For this review, take the finished solid that the model builds, in its own axes (mm). Face numbers are marked on the shaded views. A direction names the side the tool comes from. Coordinates: 2 decimals unless noted, no trailing zeros. Order: outer loops, then holes, each group sorted by start corner. A loop starts at its lowest first (then second) coordinate and runs counter-clockwise, first axis right, second up. Notation, with made-up numbers: M -16,-26 L 40,-26 A21 ccw 40,10 Z; hole C 52,32 d2. An arc over 180 degrees is marked long. Use one line per item in the form item = value. Start each with the question number.
```python
from build123d import *

# Parameters (mm, degrees)
BOSS_EXTRUDE1_DEPTH      = 8
SKETCH2_R                = 1.5
CUT_EXTRUDE1_DEPTH       = 10
SKETCH3_R                = 1.5
CUT_EXTRUDE2_DEPTH       = 10
BOSS_EXTRUDE3_DEPTH      = 30
BOSS_EXTRUDE3_DEPTH_BACK = 8
SKETCH6_W                = 20
SKETCH6_H                = 10
FILLET3_R                = 12
SKETCH7_W                = 20
SKETCH7_H                = 30
BOSS_EXTRUDE4_DEPTH      = 2
CUT_EXTRUDE3_DEPTH       = 10
SKETCH9_R                = 5.5
CUT_EXTRUDE4_DEPTH       = 10
FILLET4_R                = 5
FILLET5_R                = 2
CUT_EXTRUDE5_DEPTH       = 10
SKETCH11_W               = 20
SKETCH11_H               = 3
CUT_EXTRUDE6_DEPTH       = 15
FILLET6_R                = 2


with BuildPart() as part:
    # Sketch1 → Boss-Extrude1 (new body)
    with BuildSketch(Plane.XY):
        with BuildLine():
            Line((-25, 10), (40, 10))
            ThreePointArc((40, 10), (50, 0), (40, -10))
            Line((40, -10), (-25, -10))
            Line((-25, -10), (-25, 10))
        make_face()
    extrude(amount=BOSS_EXTRUDE1_DEPTH)

    # Sketch2 → Cut-Extrude1 (cut)
    with BuildSketch(Plane.XY.offset(8)):
        with Locations((40, 0)):
            Circle(SKETCH2_R)
    extrude(amount=-CUT_EXTRUDE1_DEPTH, mode=Mode.SUBTRACT)

    # Sketch3 → Cut-Extrude2 (cut)
    with BuildSketch(Plane(origin=(0, 0, 0), x_dir=(-1, 0, 0), z_dir=(0, 0, -1))):
        with Locations((-15, 0)):
            Circle(SKETCH3_R)
    extrude(amount=-CUT_EXTRUDE2_DEPTH, mode=Mode.SUBTRACT)

    # Sketch6 → Boss-Extrude3 (add, two sides: drawn at the far end of the back side and taken through both)
    with BuildSketch(Plane(origin=(0, 0, 0), x_dir=(-1, 0, 0), z_dir=(0, 0, -1)).offset(-BOSS_EXTRUDE3_DEPTH_BACK)):
        with Locations((15, -15)):
            Rectangle(SKETCH6_W, SKETCH6_H)
    extrude(amount=BOSS_EXTRUDE3_DEPTH + BOSS_EXTRUDE3_DEPTH_BACK)

    # Fillet3
    # the kernel refuses this fillet: 12 mm, written as the material it adds along each edge
    with BuildSketch(Plane(origin=(-5, -10, 8), x_dir=(0, -1, 0), z_dir=(0, 0, -1))) as fillet3_piece_1:
        with BuildLine():
            CenterArc((12, -11.832159566), FILLET3_R, 99.594068227, 80.405931773)
            Line((0, -11.832159566), (0, 0))
            Line((0, 0), (10, 0))
        make_face()
    extrude(amount=8)

    # Sketch7 → Boss-Extrude4 (add)
    with BuildSketch(Plane(origin=(0, -10, 0), x_dir=(1, 0, 0), z_dir=(0, 1, 0))):
        with Locations((-15, 15)):
            Rectangle(SKETCH7_W, SKETCH7_H)
    extrude(amount=BOSS_EXTRUDE4_DEPTH)

    # Sketch8 → Cut-Extrude3 (cut)
    with BuildSketch(Plane.XZ.offset(20)):
        Polygon((-12.092828782, -7.012612723), (-20.463694682, -8.488622233), (-23.370865901, -16.47600951), (-17.907171218, -22.987387277), (-9.536305318, -21.511377767), (-6.629134099, -13.52399049), align=None)
    extrude(amount=-CUT_EXTRUDE3_DEPTH, mode=Mode.SUBTRACT)

    # Sketch9 → Cut-Extrude4 (cut)
    with BuildSketch(Plane.XZ.offset(10)):
        with Locations(Location((-15, -15, 0), (0, 0, 270))):
            Circle(SKETCH9_R)
    extrude(amount=-CUT_EXTRUDE4_DEPTH, mode=Mode.SUBTRACT)

    # Fillet4
    # the kernel refuses this fillet: 5 mm, written as the material it adds along each edge
    with BuildSketch(Plane(origin=(-5, -20, 0), x_dir=(1, 0, 0), z_dir=(0, 1, 0))) as fillet4_piece_1_section:
        with BuildLine():
            CenterArc((FILLET4_R, FILLET4_R), FILLET4_R, 180, 90)
            Line((0, FILLET4_R), (0, 0))
            Line((0, 0), (FILLET4_R, 0))
        make_face()
    fillet4_piece_1 = extrude(amount=12, mode=Mode.PRIVATE)
    fillet4_piece_1 = fillet4_piece_1 - Plane(origin=(6.832159566, -22, 0), x_dir=(0, -1, 0), z_dir=(0, 0, 1)) * Cylinder(12, 44, mode=Mode.PRIVATE)
    add(fillet4_piece_1)
    with BuildSketch(Plane(origin=(-25, -8, 0), x_dir=(0, 1, 0), z_dir=(1, 0, 0))) as fillet4_piece_2:
        with BuildLine():
            CenterArc((FILLET4_R, -FILLET4_R), FILLET4_R, 90, 90)
            Line((0, -FILLET4_R), (0, 0))
            Line((0, 0), (FILLET4_R, 0))
        make_face()
    extrude(amount=20)
    with BuildSketch(Plane(origin=(-5, -20, 0), x_dir=(1, 0, 0), z_dir=(0, 1, 0))) as fillet4_piece_3a_section:
        with BuildLine():
            CenterArc((FILLET4_R, FILLET4_R), FILLET4_R, 180, 90)
            Line((0, FILLET4_R), (0, 0))
            Line((0, 0), (FILLET4_R, 0))
        make_face()
    fillet4_piece_3a = extrude(amount=24.5, mode=Mode.PRIVATE)
    fillet4_piece_3a = split(fillet4_piece_3a, bisect_by=Plane(origin=(-5, -8, 0), z_dir=(0, 1, 0)), keep=Keep.TOP, mode=Mode.PRIVATE)
    with BuildSketch(Plane(origin=(-25, -8, 0), x_dir=(0, 1, 0), z_dir=(1, 0, 0))) as fillet4_piece_3b_section:
        with BuildLine():
            CenterArc((FILLET4_R, -FILLET4_R), FILLET4_R, 90, 90)
            Line((0, -FILLET4_R), (0, 0))
            Line((0, 0), (FILLET4_R, 0))
        make_face()
    fillet4_piece_3b = extrude(amount=32.5, mode=Mode.PRIVATE)
    fillet4_piece_3b = split(fillet4_piece_3b, bisect_by=Plane(origin=(-5, -8, 0), z_dir=(1, 0, 0)), keep=Keep.TOP, mode=Mode.PRIVATE)
    fillet4_piece_3 = fillet4_piece_3a & fillet4_piece_3b
    add(fillet4_piece_3)

    # Fillet5
    fillet5_edges = [part.edges().sort_by_distance(p)[0] for p in [
        (-15, -20, 8),
        (-25, -14, -30),
        (-5, -14, -30),
        (-25, 10, 4),
    ]]
    fillet(fillet5_edges, radius=FILLET5_R)

    # Sketch10 → Cut-Extrude5 (cut)
    with BuildSketch(Plane.XY.offset(8)):
        with BuildLine():
            Line((-25, 0), (11.061986304, 10))
            Line((11.061986304, 10), (-23, 10))
            ThreePointArc((-23, 10), (-24.414213562, 9.414213562), (-25, 8))
            Line((-25, 8), (-25, 0))
        make_face()
    extrude(amount=-CUT_EXTRUDE5_DEPTH, mode=Mode.SUBTRACT)

    # Sketch11 → Cut-Extrude6 (cut)
    with BuildSketch(Plane.XZ.offset(20)):
        with Locations((-15, -28.5)):
            Rectangle(SKETCH11_W, SKETCH11_H)
    extrude(amount=-CUT_EXTRUDE6_DEPTH, mode=Mode.SUBTRACT)

    # Fillet6
    fillet6_edges = [part.edges().sort_by_distance(p)[0] for p in [
        (-25, -14, -27),
        (-5, -14, -27),
    ]]
    fillet(fillet6_edges, radius=FILLET6_R)


solid = part.part
```
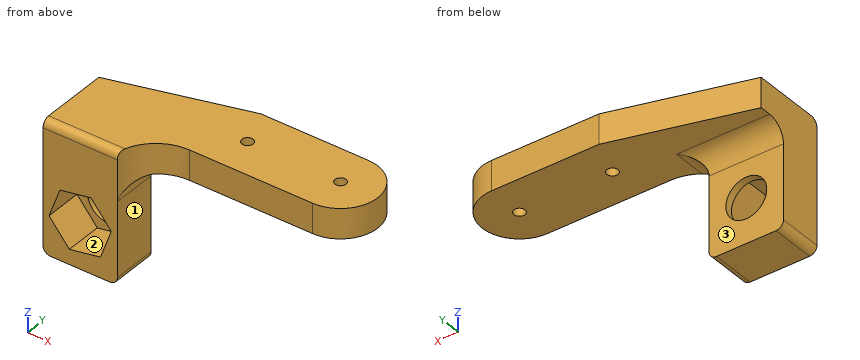
1. Tool access review of the marked faces 1, 2 and 3: name each direction out of +Z, -Z, +X, -X, +Y, -Y from which nothing blocks a thin tool from reaching the whole face with its end or side.
2. Consider section B-B, the plane z = -15. Write out the cut boundary in (x, y), plus the area to 3 significant figures.
3. Consider section C-C, the plane y = -6. Write out the cut boundary in (x, z), plus the area to 3 significant figures.
4. Consider section D-D, the plane x = -15. Write out the cut boundary in (y, z), plus the area to 3 significant figures.
5. To check wall thickness, follow line 1 (Y direction, x = 15, z = 4); line 2 (X direction, y = -9, z = -15); line 3 (Z direction, x = 29.5, y = -6). State the ranges of each line that lie inside material, in increasing order.
6. Consider section A-A, the plane x = 15. Write out the cut boundary in (y, z).
7. For pin 1 Ø10 at (x, z) = (-17.5, -12.5) entering from +Y; pin 2 Ø9 at (x, z) = (21, 5.5) entering from -Y; pin 3 Ø4 at (x, y) = (24, 6.5) entering from -Z, all flat-tipped, find the tip position at first contact; note any pin that passes through.
Answers follow:
q1.face_1 = -Z, +X, +Y, -Y
q1.face_2 = -Y
q1.face_3 = -Z, +X, -X, +Y
q2.outline = M -25,-20 L -22.83,-20 L -22.83,-10 L -20.5,-10 L -20.5,-8 L -25,-8 Z; M -9.5,-10 L -7.17,-10 L -7.17,-20 L -5,-20 L -5,-8 L -9.5,-8 Z
q2.area = 61.3 mm²
q3.outline = M -25,-1 L -3,-1 A5 cw 0,0 L 48,0 L 48,8 L -25,8 Z
q3.area = 607 mm²
q4.outline = M -20,-27 L -8,-27 L -8,-20.5 L -10,-20.5 L -10,-22.47 L -20,-22.47 Z; M -20,-7.53 L -10,-7.53 L -10,-9.5 L -8,-9.5 L -8,-5 A5 cw -3,0 L 2.77,0 L 2.77,8 L -18,8 A2 ccw -20,6 Z
q4.area = 339 mm²
q5.line_1 = -10 to -1.5, 1.5 to 10
q5.line_2 = -25 to -20.5, -9.5 to -5
q5.line_3 = 0 to 8
q6.outline = M -10,0 L -1.5,0 L -1.5,8 L -10,8 Z; M 1.5,0 L 10,0 L 10,8 L 1.5,8 Z
q7.pin_1 = -8
q7.pin_2 = -10
q7.pin_3 = 0
